from build123d import *

# Parameters (mm, degrees)
SKETCH1_W           = 45
SKETCH1_H           = 45
BOSS_EXTRUDE1_DEPTH = 3
SKETCH29_W          = 45
SKETCH29_H          = 1
BOSS_EXTRUDE2_DEPTH = 1
SKETCH30_W          = 45
SKETCH30_H          = 1
BOSS_EXTRUDE3_DEPTH = 1
CUT_EXTRUDE2_DEPTH  = 1.5
SKETCH32_W          = 12
SKETCH32_H          = 1.5
BOSS_EXTRUDE4_DEPTH = 8
SKETCH33_W          = 1
SKETCH33_H          = 0.05
CUT_EXTRUDE3_DEPTH  = 86
SKETCH34_W          = 52.951386634
SKETCH34_H          = 17.48442651
CUT_EXTRUDE4_DEPTH  = 0.1
BOSS_EXTRUDE5_DEPTH = 3
FILLET1_R           = 3


with BuildPart() as part:
    # Sketch1 → Boss-Extrude1 (new body)
    with BuildSketch(Plane(origin=(0, 0, 0), x_dir=(1, 0, 0), z_dir=(0, 1, 0))):
        Rectangle(SKETCH1_W, SKETCH1_H)
    extrude(amount=BOSS_EXTRUDE1_DEPTH)

    # Sketch29 → Boss-Extrude2 (add)
    with BuildSketch(Plane(origin=(22.5, 0, 0), x_dir=(0, 0, -1), z_dir=(1, 0, 0))):
        with Locations((0, 1.5)):
            Rectangle(SKETCH29_W, SKETCH29_H)
    extrude(amount=BOSS_EXTRUDE2_DEPTH)

    # Sketch30 → Boss-Extrude3 (add)
    with BuildSketch(Plane.ZY.offset(22.5)):
        with Locations((0, 1.5)):
            Rectangle(SKETCH30_W, SKETCH30_H)
    extrude(amount=BOSS_EXTRUDE3_DEPTH)

    # Sketch31 → Cut-Extrude2 (cut)
    with BuildSketch(Plane(origin=(0, 3, 0), x_dir=(1, 0, 0), z_dir=(0, 1, 0))):
        Polygon((-2, -22.5), (-2, -18.5), (-6, -18.5), (-6, -14.5), (6, -14.5), (6, -18.5), (2, -18.5), (2, -22.5), align=None)
    extrude(amount=-CUT_EXTRUDE2_DEPTH, mode=Mode.SUBTRACT)

    # Sketch32 → Boss-Extrude4 (add)
    with BuildSketch(Plane.XY.offset(14.5)):
        with Locations((0, 2.25)):
            Rectangle(SKETCH32_W, SKETCH32_H)
    extrude(amount=BOSS_EXTRUDE4_DEPTH)

    # Sketch33 → Cut-Extrude3 (cut)
    with BuildSketch(Plane.XY.offset(22.5)):
        with Locations((-23, 1.975)):
            Rectangle(SKETCH33_W, SKETCH33_H)
        with Locations((-23, 1.025)):
            Rectangle(SKETCH33_W, SKETCH33_H)
        with Locations((23, 1.025)):
            Rectangle(SKETCH33_W, SKETCH33_H)
        with Locations((23, 1.975)):
            Rectangle(SKETCH33_W, SKETCH33_H)
    extrude(amount=-CUT_EXTRUDE3_DEPTH, mode=Mode.SUBTRACT)

    # Sketch34 → Cut-Extrude4 (cut)
    with BuildSketch(Plane.XY.offset(22.5)):
        Rectangle(SKETCH34_W, SKETCH34_H)
    extrude(amount=-CUT_EXTRUDE4_DEPTH, mode=Mode.SUBTRACT)

    # Sketch35 → Boss-Extrude5 (add)
    with BuildSketch(Plane.XY.offset(22.4)):
        Polygon((-22.5, 3), (25.5, 3), (25.5, 0), (-25.5, 0), (-25.5, 3), align=None)
    extrude(amount=BOSS_EXTRUDE5_DEPTH)

    # Fillet1
    fillet1_edges = [part.edges().sort_by_distance(p)[0] for p in [
        (25.5, 1.5, 25.4),
        (-25.5, 1.5, 25.4),
    ]]
    fillet(fillet1_edges, radius=FILLET1_R - 0.0001)  # a hair under: the kernel refuses the full size


solid = part.part
Check sheet for the modelled part. Datum: model origin and axes. Units: mm. Round coordinates to 2 decimals unless told otherwise and drop trailing zeros. Write each loop counter-clockwise with the first axis right and the second up, starting at its lowest first coordinate (ties: lowest second). Pieces come first, ordered by that corner, then holes. Notation, with made-up numbers: (27.25, 14.25) - (86.25, 14.25) arc R5 ccw to (86.25, 23.25) - close; hole circle Ø3 at (31, 56.25). An arc over 180 degrees is marked (long way). Return JSON: item names as keys, results as strings.
Q1. Depth check by flat-ended pin: P1, Ø0.7, axis at y = 1.5, z = -9, coming from the +X side; P2, Ø0.5, axis at y = 0.5, z = -8.5, coming from the -X side; P3, Ø1, axis at y = 1.5, z = -9.5, coming from the -X side. Enter the tip coordinate at first touch or a pass-through.
Returned:
{"P1": "stops at x = 23.5", "P2": "stops at x = -22.5", "P3": "stops at x = -23.5"}
Q2. Cross-section at A-A (z = 20). Record the boundary of the cut face in (x, y).
Returned:
{"outline": "(-23.5, 1.05) - (-22.5, 1.05) - (-22.5, 0) - (22.5, 0) - (22.5, 1.05) - (23.5, 1.05) - (23.5, 1.95) - (22.5, 1.95) - (22.5, 3) - (-22.5, 3) - (-22.5, 1.95) - (-23.5, 1.95) - close"}
Q3. Scan lines: L1, parallel to X at y = 2.25, z = 13; L2, parallel to X at y = 1.65, z = -16. Record each from-to range of solid material in increasing order. Write a range as from..to.
Returned:
{"L1": "x = -22.5..22.5", "L2": "x = -23.5..23.5"}
